Geometry: final body of the model. Coordinates: model frame, mm. Face numbers are marked on the shaded views. A direction names the side the tool comes from. Give positions to 0.01 mm unless a question says otherwise; leave off trailing zeros. Write each loop counter-clockwise with the first axis right and the second up, starting at its lowest first coordinate (ties: lowest second). Pieces come first, ordered by that corner, then holes.
Q1. Pin query (flat end, axial travel): pin 1 Ø24 at (x, z) = (-56, 11) entering from +Y; pin 2 Ø3 at (x, y) = (7.5, -28) entering from +Z; pin 3 Ø5 at (y, z) = (19.5, 34.5) entering from -X. Return the tip coordinate at first contact, or that it passes through.
Q2. Mould query, pull axis Y, two halves, no side actions, for the marked faces 4, 5 and 6. Classes: +Y half, -Y half, draft (parallel to the pull), parting line (faces both ways), or undercut.
Q3. Line query: line 1 (Y direction, x = 56.5, z = 93); line 2 (X direction, y = 47.5, z = 70); line 3 (Y direction, x = -41, z = -71). Output: solid intervals per line, ascending.
Q4. Section B-B (z = -79.5). Return the cut outline in (x, y), plus the area to 3 significant figures.
Q5. Section C-C (y = 43). Return the cut outline in (x, z), plus the area to 3 significant figures.
Q6. Reachability of the marked faces 1, 2 and 3 from +Z, -Z, +X, -X, +Y, -Y: full face, straight path, thin tool, end or side. Return the list, or none.
Q7. Section D-D (z = 73). Return the cut outline in (x, y), plus the area to 3 significant figures.
Q8. Section A-A (x = 63.5). Return the cut outline in (y, z), plus the area to 3 significant figures.
from build123d import *

# Parameters (mm, degrees)
SKETCH1_W            = 80
SKETCH1_H            = 40
BOSS_EXTRUDE1_DEPTH  = 120
BOSS_EXTRUDE2_DEPTH  = 40
BOSS_EXTRUDE3_DEPTH  = 80
SKETCH1_5_W          = 80
SKETCH1_5_H          = 40
BOSS_EXTRUDE4_DEPTH  = 120
SKETCH1_6_W          = 80
SKETCH1_6_H          = 40
BOSS_EXTRUDE5_DEPTH  = 120
BOSS_EXTRUDE6_DEPTH  = 120
SKETCH1_8_W          = 80
SKETCH1_8_H          = 40
BOSS_EXTRUDE7_DEPTH  = 120
BOSS_EXTRUDE8_DEPTH  = 120
SKETCH2_W            = 80
SKETCH2_H            = 80
BOSS_EXTRUDE9_DEPTH  = 40
SKETCH3_W            = 80
SKETCH3_H            = 120
BOSS_EXTRUDE10_DEPTH = 80
SKETCH4_W            = 80
SKETCH4_H            = 40
BOSS_EXTRUDE11_DEPTH = 80


with BuildPart() as part:
    # Sketch1 → Boss-Extrude1 (new body)
    with BuildSketch(Plane.XY):
        with Locations((80, -80)):
            Rectangle(SKETCH1_W, SKETCH1_H)
    extrude(amount=BOSS_EXTRUDE1_DEPTH)

    # Sketch1<3> → Boss-Extrude2 (add)
    with BuildSketch(Plane.XY):
        Polygon((40, -100), (40, -60), (40, -20), (-120, -20), (-120, -100), align=None)
    extrude(amount=BOSS_EXTRUDE2_DEPTH)

    # Sketch1<4> → Boss-Extrude3 (add)
    with BuildSketch(Plane.XY):
        Polygon((40, -60), (120, -60), (120, 20), (40, 20), (40, -20), align=None)
    extrude(amount=BOSS_EXTRUDE3_DEPTH)

    # Sketch1<5> → Boss-Extrude4 (add)
    with BuildSketch(Plane.XY):
        with Locations((80, 40)):
            Rectangle(SKETCH1_5_W, SKETCH1_5_H)
    extrude(amount=BOSS_EXTRUDE4_DEPTH)

    # Sketch1<6> → Boss-Extrude5 (add)
    with BuildSketch(Plane.XY):
        with Locations((80, 40)):
            Rectangle(SKETCH1_6_W, SKETCH1_6_H)
    extrude(amount=-BOSS_EXTRUDE5_DEPTH)

    # Sketch1<7> → Boss-Extrude6 (add)
    with BuildSketch(Plane.XY):
        Polygon((40, -60), (120, -60), (120, 20), (40, 20), (40, -20), align=None)
    extrude(amount=-BOSS_EXTRUDE6_DEPTH)

    # Sketch1<8> → Boss-Extrude7 (add)
    with BuildSketch(Plane.XY):
        with Locations((80, -80)):
            Rectangle(SKETCH1_8_W, SKETCH1_8_H)
    extrude(amount=-BOSS_EXTRUDE7_DEPTH)

    # Sketch1<9> → Boss-Extrude8 (add)
    with BuildSketch(Plane.XY):
        Polygon((40, -100), (40, -60), (40, -20), (-120, -20), (-120, -100), align=None)
    extrude(amount=-BOSS_EXTRUDE8_DEPTH)

    # Sketch2 → Boss-Extrude9 (add)
    with BuildSketch(Plane(origin=(0, 60, 0), x_dir=(1, 0, 0), z_dir=(0, 1, 0))):
        with Locations((80, 80)):
            Rectangle(SKETCH2_W, SKETCH2_H)
    extrude(amount=BOSS_EXTRUDE9_DEPTH)

    # Sketch3 → Boss-Extrude10 (add)
    with BuildSketch(Plane.ZY.offset(-40)):
        with Locations((-80, 40)):
            Rectangle(SKETCH3_W, SKETCH3_H)
    extrude(amount=BOSS_EXTRUDE10_DEPTH)

    # Sketch4 → Boss-Extrude11 (add)
    with BuildSketch(Plane.ZY.offset(40)):
        with Locations((-80, 0)):
            Rectangle(SKETCH4_W, SKETCH4_H)
    extrude(amount=BOSS_EXTRUDE11_DEPTH)


solid = part.part
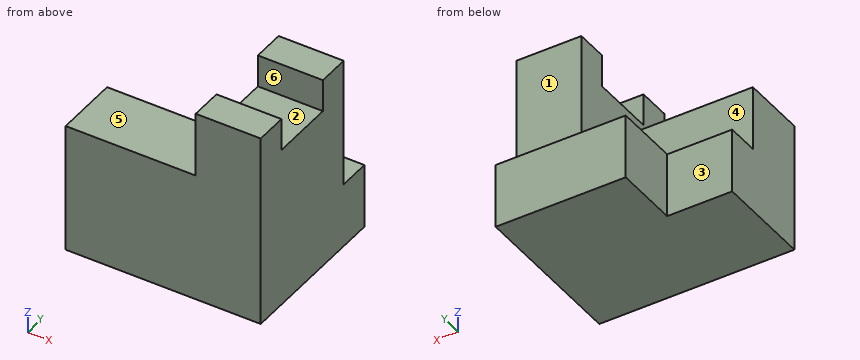
Computed:
1. pin 1: stops at y = -20
1. pin 2: stops at z = 40
1. pin 3: stops at x = 40
2. face 4: +Y half
2. face 5: draft
2. face 6: undercut
3. line 1: y = -100 to -60, 20 to 60
3. line 2: x = 40 to 120
3. line 3: y = -100 to 20
4. outline: (-120, -100) - (120, -100) - (120, 100) - (-40, 100) - (-40, 20) - (-120, 20) - close
4. area: 41,600 mm2
5. outline: (-40, -120) - (120, -120) - (120, 120) - (40, 120) - (40, -40) - (-40, -40) - close
5. area: 25,600 mm2
6. face 1: +Z, +X, -X, +Y
6. face 2: +Z, +X, -X
6. face 3: +Z, -Z, -X, +Y
7. outline: (40, -100) - (120, -100) - (120, 60) - (40, 60) - close
7. area: 12,800 mm2
8. outline: (-100, -120) - (100, -120) - (100, -40) - (60, -40) - (60, 120) - (20, 120) - (20, 80) - (-60, 80) - (-60, 120) - (-100, 120) - close
8. area: 38,400 mm2
